Geometry check sheet. Reference: the model listing, model coordinates, mm. Face numbers are marked on the shaded views. A direction names the side the tool comes from. Round coordinates to 2 decimals unless told otherwise and drop trailing zeros. Write each loop counter-clockwise with the first axis right and the second up, starting at its lowest first coordinate (ties: lowest second). Pieces come first, ordered by that corner, then holes. Notation, with made-up numbers: (52, -37) -> (91, -37) arc R7 ccw to (91, -28) -> close; hole circle Ø6 at (34.25, -18.75). An arc over 180 degrees is marked (long way). Use a Markdown table: item, result.
Autodesk Inventor part; units mm, degrees
ref_plane "Work Plane1" through (-100, 0, 27.5) normal (0, 0, 1) x (1, 0, 0)
ref_plane "YZ Plane" through (0, 0, 0) normal (1, 0, 0) x (0, 1, 0)
ref_plane "XZ Plane" through (0, 0, 0) normal (0, 1, 0) x (-1, 0, 0)
sketch "Sketch1" plane through (0, 0, 0) normal (0, 1, 0) x (-1, 0, 0)
  line L0 (0, 0) -> (100, 0)
  line L1 (100, 0) -> (100, 55)
  line L2 (100, 55) -> (0, 55)
  line L3 (0, 55) -> (0, 0)
  dimension "d0" = 55
  dimension "d1" = 100
extrude "Extrusion1" add sketch "Sketch1" along normal blind 40
sketch "Sketch2" plane through (0, 0, 0) normal (0, -1, 0) x (1, 0, 0)
  circle A0 centre (-5, 3.75) radius 2.5
  line L0 (0, 55) -> (0, 0)
  line L1 (0, 0) -> (-100, 0)
  line L2 (0, 0) -> (-100, 0)
  line L3 (-50, 0) -> (-50, 13.5836)
  line L4 (0, 55) -> (0, 0)
  line L5 (0, 27.5) -> (-21.4459, 27.5)
  circle A1 centre (-5, 51.25) radius 2.5
  circle A2 centre (-95, 3.75) radius 2.5
  circle A3 centre (-95, 51.25) radius 2.5
  dimension "d4" = 5
  dimension "d5" = 5
  dimension "d6" = 3.75
extrude "Extrusion2" cut sketch "Sketch2" against normal blind 18
sketch "Sketch3" plane through (0, 0, 0) normal (0, -1, 0) x (1, 0, 0)
  line L0 (-97.5, 7.5) -> (-10, 7.5)
  line L1 (-10, 7.5) -> (-10, 47.5)
  line L2 (-10, 47.5) -> (-97.5, 47.5)
  line L3 (-97.5, 47.5) -> (-97.5, 7.5)
  line L4 (-100, 0) -> (-100, 55)
  line L5 (-100, 55) -> (0, 55)
  point P0 (0, 0)
  dimension "d9" = 2.5
  dimension "d10" = 87.5
  dimension "d11" = 40
  dimension "d12" = 55
  dimension "d13" = 7.5
extrude "Extrusion3" cut sketch "Sketch3" against normal blind 10
sketch "Sketch4" plane through (0, 10, 0) normal (0, -1, 0) x (1, 0, 0)
  line L0 (-10, 47.5) -> (-10, 7.5)
  line L1 (-97.5, 47.5) -> (-10, 47.5)
  line L2 (-10, 7.5) -> (-75, 7.5)
  line L3 (-75, 7.5) -> (-75, 47.5)
  line L4 (-75, 47.5) -> (-10, 47.5)
  line L5 (-10, 47.5) -> (-10, 7.5)
  point P0 (0, 0)
  dimension "d16" = 65
extrude "Extrusion4" cut sketch "Sketch4" against normal through all
sketch "Sketch5" plane through (0, 0, 55) normal (1, 0, 0) x (0, 0, -1)
  circle A0 centre (27.5, 16) radius 5
  line L0 (55, 0) -> (55, 40)
  line L1 (0, 0) -> (0, 40)
  line L2 (0, 0) -> (55, 0)
  dimension "d19" = 27.5
  dimension "d20" = 55
  dimension "d21" = 10
  dimension "d22" = 16
extrude "Extrusion5" cut sketch "Sketch5" against normal through all
sketch "Sketch6" plane through (0, 0, 55) normal (1, 0, 0) x (0, 0, -1)
  circle A0 centre (27.5, 16) radius 5
  circle A1 centre (27.5, 16) radius 7.5
  point P0 (55, 0)
  dimension "d25" = 15
extrude "Extrusion6" cut sketch "Sketch6" against normal blind 1
sketch "Sketch7" plane through (-100, 0, 0) normal (-1, 0, 0) x (0, 0, 1)
  circle A0 centre (27.5, 16) radius 5
  circle A1 centre (27.5, 16) radius 7.5
  point P0 (0, 0)
  dimension "d28" = 15
extrude "Extrusion7" cut sketch "Sketch7" against normal blind 1
sketch "Sketch8" plane through (-100, 0, 55) normal (0, 0, 1) x (1, 0, 0)
  circle A0 centre (80, 15) radius 2.5
  line L0 (100, 0) -> (100, 40)
  line L1 (0, 0) -> (100, 0)
  circle A1 centre (20, 15) radius 2.5
  line L2 (0, 0) -> (0, 40)
  dimension "d31" = 5
  dimension "d32" = 20
  dimension "d33" = 15
  dimension "d34" = 5
  dimension "d35" = 20
  dimension "d36" = 15
extrude "Extrusion8" cut sketch "Sketch8" against normal blind 15
ref_plane "Work Plane1" through (-100, 0, 27.5) normal (0, 0, 1) x (1, 0, 0)
mirror "Mirror1" about plane through (-100, 0, 27.5) normal (0, 0, 1) of "Extrusion8"
fillet "Fillet1" radius 5 6 edges at (-97.5, 5, 7.5) (-97.5, 5, 47.5) (-10, 20, 7.5) (-10, 20, 47.5) (-75, 25, 7.5) (-75, 25, 47.5)
sketch "Sketch10" plane through (0, 40, 0) normal (0, 1, 0) x (1, 0, 0)
  arc A0 (-78, -48) -> (-86, -48) centre (-82, -48) ccw
  line L0 (-78, -48) -> (-78, -67.7659)
  line L1 (-78, -67.7659) -> (-86, -67.7659)
  line L2 (-86, -67.7659) -> (-86, -48)
  line L3 (-100, -55) -> (0, -55)
  line L4 (-100, 0) -> (-100, -55)
  arc A1 (-3, -48) -> (-11, -48) centre (-7, -48) ccw
  line L5 (-3, -48) -> (-3, -67.2517)
  line L6 (-3, -67.2517) -> (-11, -67.2517)
  line L7 (-11, -67.2517) -> (-11, -48)
  line L8 (0, -55) -> (0, 0)
  line L9 (-100, 0) -> (-100, -55)
  line L10 (-100, -27.5) -> (-88.5894, -27.5)
  arc A2 (-86, -7) -> (-78, -7) centre (-82, -7) ccw
  line L11 (-78, -7) -> (-78, 12.7659)
  line L12 (-78, 12.7659) -> (-86, 12.7659)
  line L13 (-86, 12.7659) -> (-86, -7)
  line L14 (-100, 0) -> (0, 0)
  arc A3 (-11, -7) -> (-3, -7) centre (-7, -7) ccw
  line L15 (-3, -7) -> (-3, 12.2517)
  line L16 (-3, 12.2517) -> (-11, 12.2517)
  line L17 (-11, 12.2517) -> (-11, -7)
  dimension "d40" = 8
  dimension "d41" = 7
  dimension "d43" = 8
  dimension "d44" = 7
  dimension "d45" = 7
  dimension "d48" = 82
extrude "Extrusion9" cut sketch "Sketch10" against normal blind 8 contours L0 L3 L2 A0 | L0 L1 L2 L3 | L7 A1 L5 L3 | L3 L5 L6 L7 | L14 L11 A2 L13 | L13 L12 L11 L14 | L15 A3 L17 L14 | L14 L17 L16 L15
sketch "Sketch11" plane through (0, 0, 0) normal (-1, 0, 0) x (0, 0, 1)
  circle A0 centre (5.5, 34.5) radius 2
  line L0 (0, 40) -> (55, 40)
  line L1 (0, 0) -> (0, 40)
  line L2 (55, 40) -> (0, 40)
  line L3 (27.5, 40) -> (27.5, 46.5712)
  circle A1 centre (49.5, 34.5) radius 2
  dimension "d49" = 4
  dimension "d50" = 5.5
  dimension "d51" = 5.5
extrude "Extrusion10" cut sketch "Sketch11" along normal blind 13
sketch "Sketch12" plane through (0, 40, 0) normal (0, 1, 0) x (1, 0, 0)
  line L0 (-100, -55) -> (0, -55)
  line L1 (0, 0) -> (-100, 0)
  line L2 (-100, -55) -> (-89, -55)
  line L3 (-89, -55) -> (-89, 0)
  line L4 (-89, 0) -> (-100, 0)
  line L5 (-100, 0) -> (-100, -55)
  line L6 (-86, -55) -> (-86, -48)
  dimension "d54" = 3
extrude "Extrusion11" cut sketch "Sketch12" against normal blind 13
sketch "Sketch13" plane through (-89, 40, 0) normal (-1, 0, 0) x (0, 0, 1)
  circle A0 centre (5.5, -5.5) radius 2
  circle A1 centre (49.5, -5.5) radius 2
  point P0 (0, -40)
extrude "Extrusion12" cut sketch "Sketch13" against normal blind 13
sketch "Sketch15" plane through (-89, 40, 0) normal (-1, 0, 0) x (0, 0, 1)
  circle A0 centre (27.5, 15) radius 22
  line L0 (0, -13) -> (0, 0)
  line L1 (0, 0) -> (55, 0)
  point P0 (0, -40)
  dimension "d59" = 27.5
  dimension "d60" = 15
  dimension "d61" = 44
extrude "Extrusion13" cut sketch "Sketch15" against normal through all
equation "\"d13\" = -0.5 * d11 + 0.5 * d12"
equation "\"d19\" = 0.5 * d20"
equation "\"d36\" = d33"
equation "\"d51\" = d50"
properties part number "CarterRouleau" material "Aluminum 6061"
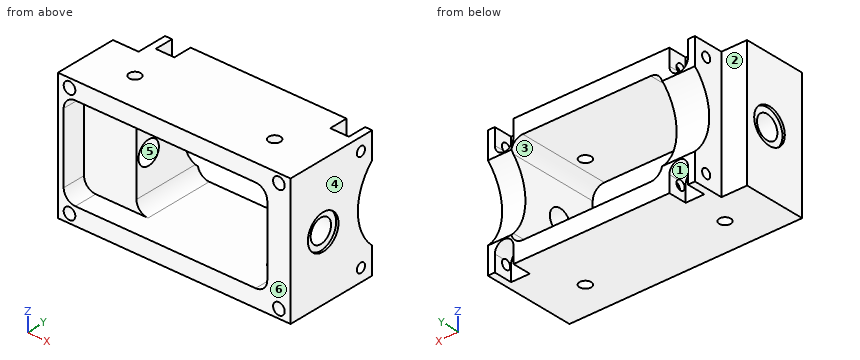
(1) Thickness scan on line 1 (X direction, y = 33.5, z = 52); line 2 (Z direction, x = -71.5, y = 5); line 3 (Y direction, x = -80, z = 50). Record the ranges inside material, lowest first.
A:
| item | result |
|---|---|
| line 1 | x = -89 to -86, -78 to -11, -3 to 0 |
| line 2 | z = 0 to 7.5, 47.5 to 55 |
| line 3 | y = 0 to 12.5, 17.5 to 32 |
(2) Access from +Z, -Z, +X, -X, +Y, -Y to the whole of each face (thin tool, end or side, straight path). Record for the marked faces 1, 2 and 3.
A:
| item | result |
|---|---|
| face 1 | -Z, +Y |
| face 2 | +Z, -Z, -X, +Y |
| face 3 | +Y, -Y |
(3) Section check D-D on z = 25.5. Record the cut outline in (x, y).
A:
| item | result |
|---|---|
| outline | (-100, 0) -> (-97.5, 0) -> (-97.5, 10) -> (-75, 10) -> (-75, 11.42) -> (-99, 11.42) -> (-99, 8.77) -> (-100, 8.77) -> close; (-100, 23.23) -> (-99, 23.23) -> (-99, 20.58) -> (-75, 20.58) -> (-75, 33.09) -> (-89, 33.09) -> (-89, 27) -> (-100, 27) -> close; (-10, 0) -> (0, 0) -> (0, 8.77) -> (-1, 8.77) -> (-1, 11.42) -> (-10, 11.42) -> close; (-10, 20.58) -> (-1, 20.58) -> (-1, 23.23) -> (0, 23.23) -> (0, 33.09) -> (-10, 33.09) -> close |
(4) Section check B-B on y = 5. Record the cut outline in (x, z).
A:
| item | result |
|---|---|
| outline | (-100, 0) -> (0, 0) -> (0, 55) -> (-100, 55) -> close; hole circle Ø5 at (-95, 3.75); hole (-97.5, 12.5) arc R5 ccw to (-92.5, 7.5) -> (-15, 7.5) arc R5 ccw to (-10, 12.5) -> (-10, 42.5) arc R5 ccw to (-15, 47.5) -> (-92.5, 47.5) arc R5 ccw to (-97.5, 42.5) -> close; hole circle Ø5 at (-95, 51.25); hole circle Ø5 at (-5, 3.75); hole circle Ø5 at (-5, 51.25) |
(5) Release check for a two-part mould opening along Y. For the marked faces 4, 5 and 6 record: +Y half, -Y half, draft (parallel to the pull), parting line (faces both ways), or undercut.
A:
| item | result |
|---|---|
| face 4 | draft |
| face 5 | undercut |
| face 6 | -Y half |
(6) Section check C-C on x = -80. Record the cut outline in (y, z), plus the area to 3 significant figures.
A:
| item | result |
|---|---|
| outline | (0, 0) -> (12.5, 0) -> (12.5, 15) -> (17.5, 15) -> (17.5, 0) -> (32, 0) -> (32, 10.46) -> (40, 10.46) -> (40, 11.41) arc R22 cw to (40, 43.59) -> (40, 44.54) -> (32, 44.54) -> (32, 55) -> (17.5, 55) -> (17.5, 40) -> (12.5, 40) -> (12.5, 55) -> (0, 55) -> (0, 47.5) -> (10, 47.5) -> (10, 7.5) -> (0, 7.5) -> close; hole circle Ø10 at (16, 27.5) |
| area | 1,250 mm2 |
(7) Section check A-A on y = 28.5. Record the cut outline in (x, z).
A:
| item | result |
|---|---|
| outline | (-89, 0) -> (0, 0) -> (0, 55) -> (-89, 55) -> close; hole (-75, 12.5) arc R5 ccw to (-70, 7.5) -> (-15, 7.5) arc R5 ccw to (-10, 12.5) -> (-10, 42.5) arc R5 ccw to (-15, 47.5) -> (-70, 47.5) arc R5 ccw to (-75, 42.5) -> close |
(8) Gauge pin test, flat ends, axial feed: pin 1 Ø3 at (y, z) = (33.5, 20) entering from -X; pin 2 Ø4 at (x, z) = (-7.5, 47.5) entering from +Y; pin 3 Ø6.5 at (x, z) = (-95, 51.25) entering from +Y. Record the tip position at first contact, or that the pin passes through.
A:
| item | result |
|---|---|
| pin 1 | stops at x = -89 |
| pin 2 | stops at y = 32 |
| pin 3 | stops at y = 27 |
